Source: three-view drawing plus pictorial views. Frame: mm from the lowest corner of the part. Give positions to 0.01 mm unless a question says otherwise; leave off trailing zeros. Order: outer loops, then holes, each group sorted by start corner. A loop starts at its lowest first (then second) coordinate and runs counter-clockwise, first axis right, second up. Notation, with made-up numbers: (63, -7.75) - (105, -7.75) arc R20 cw to (105, 14.25) - close; hole circle Ø2 at (12.25, 61.5). An arc over 180 degrees is marked (long way). Use CSV: the item, a comma, the result in double quotes.
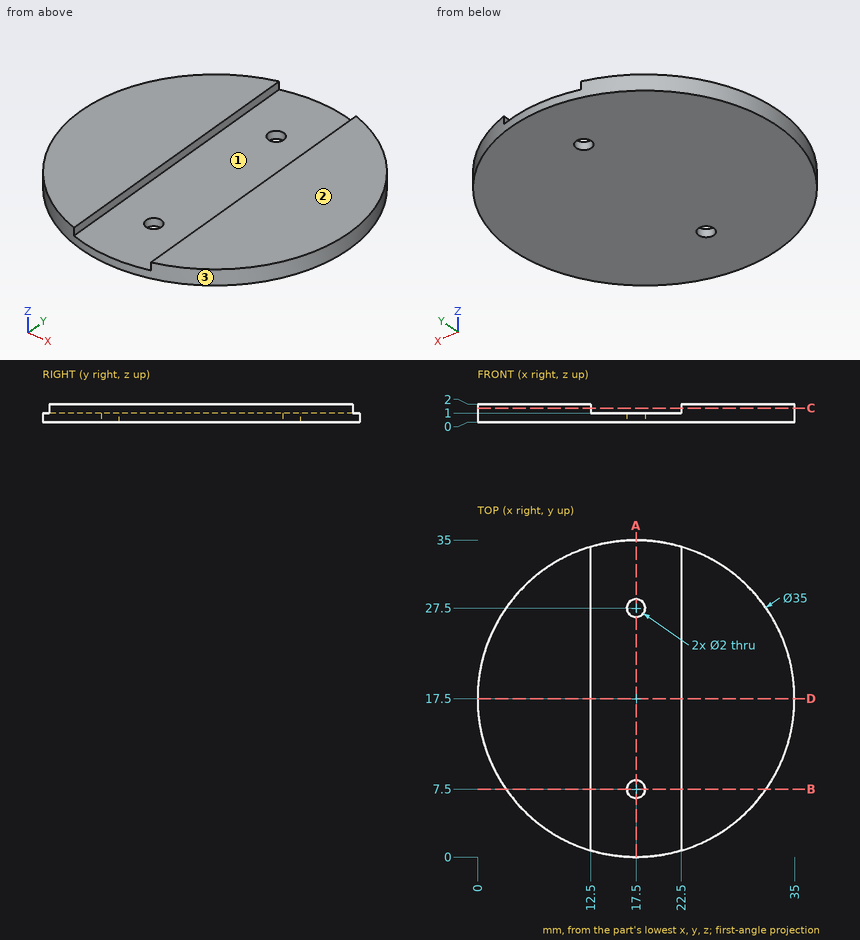
Item 1: Section A-A on x = 17.5. Return the cut outline in (y, z).
Filled in:
outline,"(0, 0) - (6.5, 0) - (6.5, 1) - (0, 1) - close; (8.5, 0) - (26.5, 0) - (26.5, 1) - (8.5, 1) - close; (28.5, 0) - (35, 0) - (35, 1) - (28.5, 1) - close"
Item 2: First-contact query: pin 1 (6 mm diameter, centred on x = 16, y = 22, fed in from -Z); pin 2 (1.1 mm diameter, centred on y = 12, z = 1.5, fed in from -X); pin 3 (3 mm diameter, centred on x = 17.5, y = 27.5, fed in from +Z); pin 4 (1.8 mm diameter, centred on x = 17.5, y = 7.5, fed in from +Z). Flat tips, straight axial feed; report the tip coordinate or a pass-through.
Filled in:
pin 1,"stops at z = 0"
pin 2,"stops at x = 0.71"
pin 3,"stops at z = 1"
pin 4,"passes through"
Item 3: Material intervals for line 1 (Y direction, x = 17.5, z = 0.1); line 2 (X direction, y = 12.5, z = 1.85); line 3 (X direction, y = 7.5, z = 0.6), sorted ascending. Write a range as from..to.
Filled in:
line 1,"y = 0..6.5, 8.5..26.5, 28.5..35"
line 2,"x = 0.73..12.5, 22.5..34.27"
line 3,"x = 3.14..16.5, 18.5..31.86"
Item 4: Mould query, pull axis X, two halves, no side actions, for the marked faces 1, 2 and 3. Classes: released by +X, released by -X, zero draft, split by the parting line, or undercut.
Filled in:
face 1,"undercut"
face 2,"zero draft"
face 3,"split by the parting line"
Item 5: Section D-D on y = 17.5. Return the cut outline in (x, z).
Filled in:
outline,"(0, 0) - (35, 0) - (35, 2) - (22.5, 2) - (22.5, 1) - (12.5, 1) - (12.5, 2) - (0, 2) - close"
Item 6: Section B-B on y = 7.5. Return the cut outline in (x, z), then the cut area to 3 significant figures.
Filled in:
outline,"(3.14, 0) - (16.5, 0) - (16.5, 1) - (12.5, 1) - (12.5, 2) - (3.14, 2) - close; (18.5, 0) - (31.86, 0) - (31.86, 2) - (22.5, 2) - (22.5, 1) - (18.5, 1) - close"
area,"45.4 mm2"
Item 7: Section C-C on z = 1.55. Return the cut outline in (x, y), then the cut area to 3 significant figures.
Filled in:
outline,"(12.5, 0.73) - (12.5, 34.27) arc R17.5 ccw to start; (22.5, 0.73) arc R17.5 ccw to (22.5, 34.27) - close"
area,"617 mm2"
